Geometry: see drawing. Coordinates: mm, zero at the bounding-box minimum. Round coordinates to 2 decimals unless told otherwise and drop trailing zeros. Order: outer loops, then holes, each group sorted by start corner. A loop starts at its lowest first (then second) coordinate and runs counter-clockwise, first axis right, second up. Notation, with made-up numbers: (9.5, -23.5) -> (17.5, -23.5) arc R28 ccw to (17.5, -4.5) -> close; hole circle Ø1 at (63.25, 30). An arc over 180 degrees is marked (long way). Use a Markdown table: item, result.
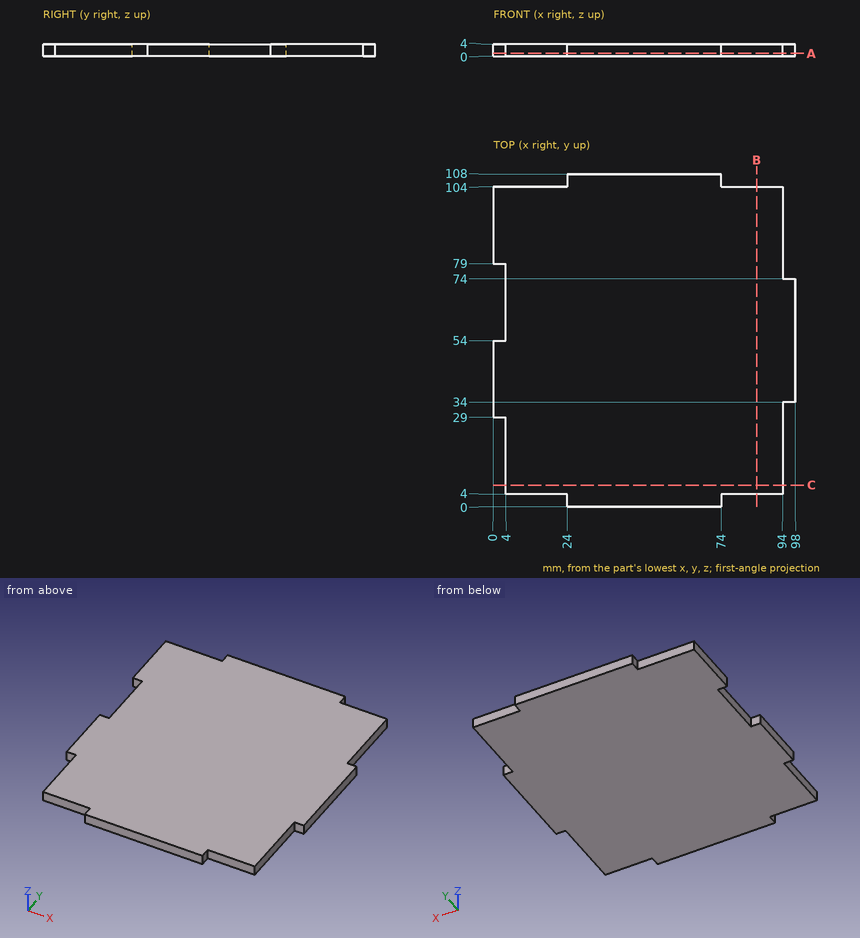
1) Ray query, probe 1 along Y at (x, z) = (88, 2.2); probe 2 along X at (y, z) = (6, 0.45); probe 3 along X at (y, z) = (67, 3.6). Return the intervals inside material, ascending.
Answer key:
| item | result |
|---|---|
| probe 1 | y = 4 to 104 |
| probe 2 | x = 4 to 94 |
| probe 3 | x = 4 to 98 |
2) Cut plane C-C on y = 7. Return loops of the section in (x, z).
Answer key:
| item | result |
|---|---|
| outline | (4, 0) -> (94, 0) -> (94, 4) -> (4, 4) -> close |
3) Cut plane A-A on z = 0.95. Return loops of the section in (x, y), and give its area (3 significant figures).
Answer key:
| item | result |
|---|---|
| outline | (0, 29) -> (4, 29) -> (4, 4) -> (24, 4) -> (24, 0) -> (74, 0) -> (74, 4) -> (94, 4) -> (94, 34) -> (98, 34) -> (98, 74) -> (94, 74) -> (94, 104) -> (74, 104) -> (74, 108) -> (24, 108) -> (24, 104) -> (0, 104) -> (0, 79) -> (4, 79) -> (4, 54) -> (0, 54) -> close |
| area | 9,760 mm^2 |
4) Contact query for flat-ended pins moving along their axis: P1, Ø2, axis at y = 22, z = 1, coming from the +X side; P2, Ø2, axis at x = 3, z = 1.5, coming from the +Y side; P3, Ø1, axis at x = 11, z = 3.5, coming from the -Y side. Output: stop coordinate, or through.
Answer key:
| item | result |
|---|---|
| P1 | stops at x = 94 |
| P2 | stops at y = 104 |
| P3 | stops at y = 4 |
5) Cut plane B-B on x = 85.5. Return loops of the section in (y, z).
Answer key:
| item | result |
|---|---|
| outline | (4, 0) -> (104, 0) -> (104, 4) -> (4, 4) -> close |
